The figure shows three views and two pictorial views of one solid part (mm, origin at its lowest corner). Answer the questions. A direction names the side the tool comes from. Give positions to 0.01 mm unless a question says otherwise; leave off trailing zeros. Write each loop counter-clockwise with the first axis right and the second up, starting at its lowest first coordinate (ties: lowest second). Pieces come first, ordered by that corner, then holes. Notation, with made-up numbers: M 88.25,85 L 94.25,85 A30 ccw 94.25,118 Z; hole C -22,72.25 d3. An arc over 180 degrees is marked long. Return JSON: item names as keys, results as strings.
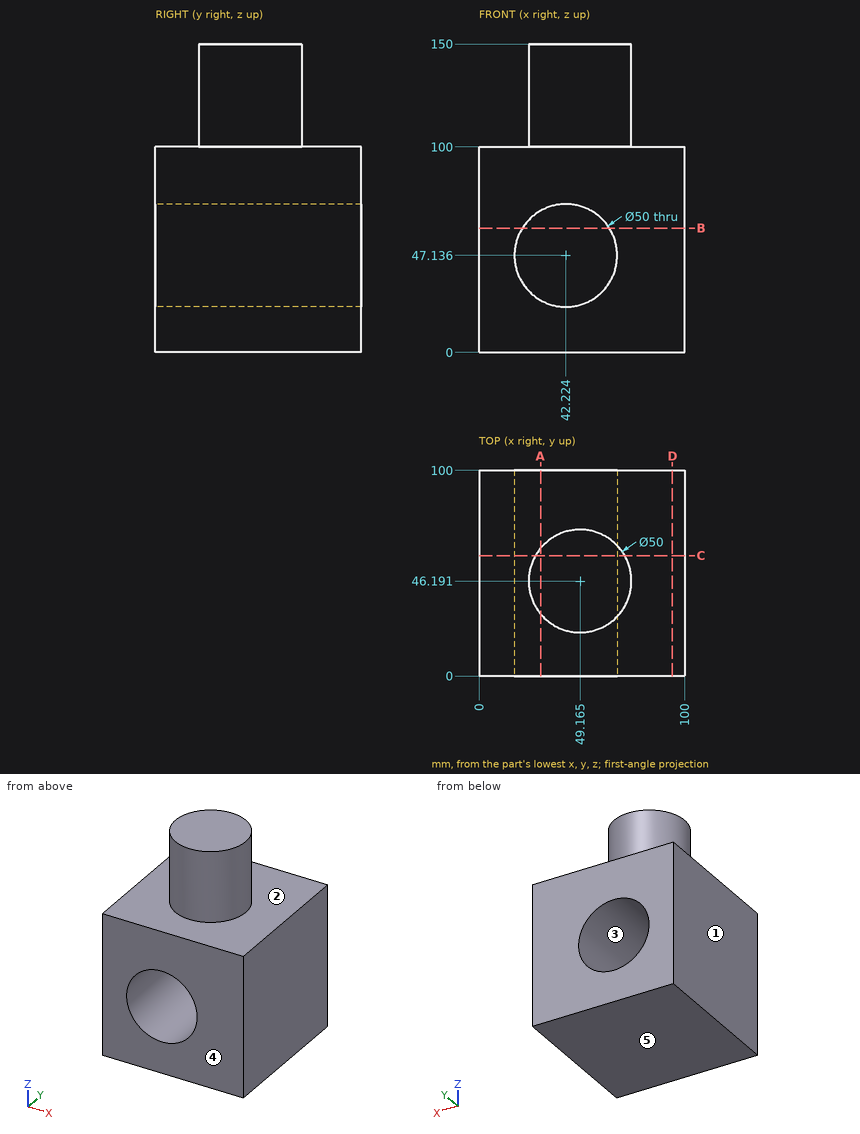
Item 1: Which of the six approach directions +Z, -Z, +X, -X, +Y, -Y give full straight-line access (tool end or side, diameter ignored) to the marked faces 1 and 2?
Geometry results:
{"face 1": "+Z, -Z, -X, +Y, -Y", "face 2": "+Z"}
Item 2: A cutting plane is placed at D-D, the plane x = 94. Write down the section's boundary in (y, z), plus the area to 3 significant figures.
Geometry results:
{"outline": "M 0,0 L 100,0 L 100,100 L 0,100 Z", "area": "10,000 mm2"}
Item 3: A cutting plane is placed at B-B, the plane z = 60.5. Write down the section's boundary in (x, y), plus the area to 3 significant figures.
Geometry results:
{"outline": "M 0,0 L 21.1,0 L 21.1,100 L 0,100 Z; M 63.35,0 L 100,0 L 100,100 L 63.35,100 Z", "area": "5,770 mm2"}
Item 4: A cutting plane is placed at C-C, the plane y = 58.5. Write down the section's boundary in (x, z) (1 decimal), plus the area to 3 significant figures.
Geometry results:
{"outline": "M 0,0 L 100,0 L 100,100 L 70.9,100 L 70.9,150 L 27.4,150 L 27.4,100 L 0,100 Z; hole C 42.2,47.1 d50", "area": "10,200 mm2"}
Item 5: A cutting plane is placed at A-A, the plane x = 30. Write down the section's boundary in (y, z), plus the area to 3 significant figures.
Geometry results:
{"outline": "M 0,0 L 100,0 L 100,25.33 L 0,25.33 Z; M 0,68.94 L 100,68.94 L 100,100 L 62.24,100 L 62.24,150 L 30.14,150 L 30.14,100 L 0,100 Z", "area": "7,240 mm2"}
Item 6: Determine the mould class of the marked faces 3, 4 and 5 for opening direction Z: +Z half, -Z half, draft (parallel to the pull), parting line (faces both ways), or undercut.
Geometry results:
{"face 3": "undercut", "face 4": "draft", "face 5": "-Z half"}
Item 7: Find the intervals of material crossed by line 1 (Z direction, x = 41, y = 26) (1 decimal); line 2 (Z direction, x = 89.5, y = 11.5); line 3 (X direction, y = 74, z = 56.5) (1 decimal), in increasing order.
Geometry results:
{"line 1": "z = 0 to 22.2, 72.1 to 150", "line 2": "z = 0 to 100", "line 3": "x = 0 to 19, 65.4 to 100"}
